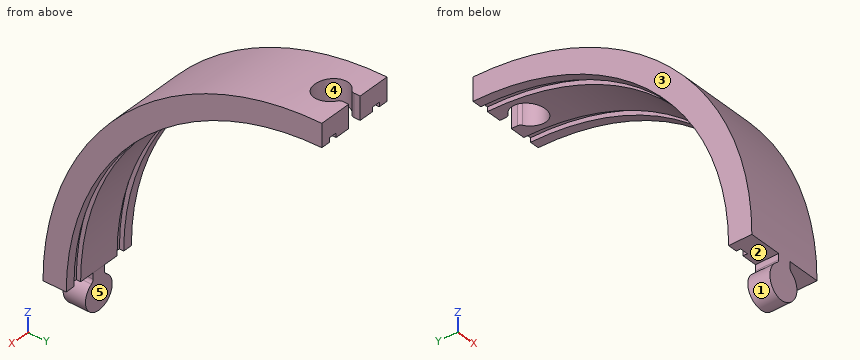
Autodesk Inventor part; units mm, degrees
ref_plane "YZ Plane" through (0, 0, 0) normal (1, 0, 0) x (0, 1, 0)
ref_plane "XZ Plane" through (0, 0, 0) normal (0, 1, 0) x (-1, 0, 0)
ref_plane "XY Plane" through (0, 0, 0) normal (0, 0, 1) x (1, 0, 0)
sketch "Track sketch" plane through (0, 0, 0) normal (0, 0, 1) x (1, 0, 0)
  line L0 (0, 0) -> (86.36, 0)
  line L1 (86.36, 0) -> (86.36, 25.4)
  line L2 (0, 25.4) -> (0, 0)
  line L3 (19.05, 25.4) -> (19.05, 20.6375)
  line L4 (19.05, 20.6375) -> (10.16, 20.6375)
  line L5 (10.16, 20.6375) -> (10.16, 25.4)
  line L6 (43.18, 25.4) -> (43.18, 0) construction
  line L7 (67.31, 25.4) -> (67.31, 20.6375)
  line L8 (67.31, 20.6375) -> (76.2, 20.6375)
  line L9 (76.2, 20.6375) -> (76.2, 25.4)
  line L10 (10.16, 25.4) -> (0, 25.4)
  line L11 (86.36, 25.4) -> (76.2, 25.4)
  line L12 (67.31, 25.4) -> (19.05, 25.4)
  line L13 (0, 0) -> (0, 304.8) construction
  line L14 (0, 304.8) -> (86.36, 304.8) construction
  line L15 (0, 0) -> (0, -25.4)
  line L16 (0, -25.4) -> (86.36, -25.4)
  line L17 (86.36, -25.4) -> (86.36, 0)
  dimension "d0" = 86.36
  dimension "d1" = 25.4
  dimension "d2" = 19.05
  dimension "d3" = 10.16
  dimension "d6" = 4.7625
  dimension "d23" = 304.8
  dimension "d47" = 25.4
revolve "Revolution1" add sketch "Track sketch" angle 90 about axis through (0, 304.8, 0) along (-1, 0, 0) contours L2 L10 L5 L4 L3 L12 L7 L8 L9 L11 L1 L0
sketch "Sketch3" plane through (0, 0, 0) normal (0, 1, 0) x (-1, 0, 0)
  line L0 (-19.50225, 0) -> (-66.85775, 0)
  line L1 (-43.18, 304.8) -> (-43.18, 0) construction
  line L2 (-43.18, 0) -> (-43.18, -37.562444) construction
  arc A0 (-52.968989, -10.557355) -> (-33.391011, -10.557355) centre (-43.18, -25.4) ccw
  line L3 (-50.8, 0) -> (-35.56, 0)
  line L4 (-35.56, 0) -> (-35.56, -6.528638)
  line L5 (-35.56, -9.335629) -> (-50.8, -9.335629) construction
  line L6 (-50.8, -6.528638) -> (-50.8, 0)
  arc A1 (-52.968989, -10.557355) -> (-50.8, -6.528638) centre (-55.626, -6.528638) ccw
  arc A2 (-35.56, -6.528638) -> (-33.391011, -10.557355) centre (-30.734, -6.528638) ccw
  line L7 (0, 0) -> (-86.36, 0)
  line L8 (-86.36, 0) -> (-86.36, 304.8)
  line L9 (0, 304.8) -> (-86.36, 304.8)
  line L10 (0, 0) -> (0, 304.8)
  line L11 (0, 0) -> (-86.36, 0)
  line L12 (0, 304.8) -> (-86.36, 304.8) construction
  line L13 (-43.18, 304.8) -> (-43.18, 65.498651) construction
  point P0 (-43.18, 279.4)
  dimension "d25" = 279.4
  dimension "d26" = 35.56
  dimension "d27" = 25.4
  dimension "d28" = 15.24
  dimension "d29" = 4.826
  dimension "d32" = 86.36
  dimension "d33" = 43.18
  dimension "d34" = 43.18
  dimension "d35" = 25.4
extrude "Extrusion4" add sketch "Sketch3" along normal blind 25.4 contours L4 A2 A0 A1 L6 L0
ref_plane "Work Plane1" through (0, 304.8, 304.8) normal (0, 0, 1) x (1, 0, 0)
sketch "Sketch4" plane through (0, 304.8, 304.8) normal (0, 0, 1) x (1, 0, 0)
  line L0 (0, -304.8) -> (35.56, -304.8)
  line L1 (35.56, -304.8) -> (50.8, -304.8)
  line L2 (50.8, -304.8) -> (86.36, -304.8)
  line L3 (86.36, -304.8) -> (86.36, 0)
  line L4 (0, 0) -> (86.36, 0)
  line L5 (0, -304.8) -> (0, 0)
  line L6 (67.31, 0) -> (19.05, 0)
  line L7 (43.18, 304.8) -> (43.18, 0) construction
  line L8 (43.18, 0) -> (43.18, -37.562444) construction
  arc A0 (33.391011, -10.557355) -> (52.968989, -10.557355) centre (43.18, -25.4) ccw
  line L9 (35.56, 0) -> (50.8, 0)
  line L10 (50.8, 0) -> (50.8, -6.528638)
  line L11 (50.8, -9.335629) -> (35.56, -9.335629) construction
  line L12 (35.56, -6.528638) -> (35.56, 0)
  arc A1 (33.391011, -10.557355) -> (35.56, -6.528638) centre (30.734, -6.528638) ccw
  arc A2 (50.8, -6.528638) -> (52.968989, -10.557355) centre (55.626, -6.528638) ccw
  point P0 (43.18, 279.4)
  dimension "d38" = 279.4
  dimension "d39" = 35.56
  dimension "d40" = 25.4
  dimension "d41" = 15.24
  dimension "d42" = 4.826
  dimension "d43" = 43.18
  dimension "d44" = 25.4
extrude "Extrusion5" cut sketch "Sketch4" against normal blind 50.8 contours L4 L10 A2 A0 A1 L12
sketch "Track sketch outline for Revolution2" plane through (0, 0, 0) normal (0, 0, 1) x (1, 0, 0)
  line L0 (86.36, 0) -> (0, 0)
  line L1 (86.36, -25.4) -> (86.36, 0)
  line L2 (0, -25.4) -> (86.36, -25.4)
  line L3 (0, 0) -> (0, -25.4)
revolve "Revolution2" cut sketch "Track sketch outline for Revolution2" angle 360 about axis through (0, 304.8, 0) along (1, 0, 0)
properties part number "Caufield_Straight_Track"
Part model, mm, in its own coordinate system. Face numbers are marked on the shaded views. A direction names the side the tool comes from. Coordinates: 2 decimals unless noted, no trailing zeros. Loops run counter-clockwise (first coordinate to the right, second up) from the corner with the lowest first, then second, coordinate; pieces in that order, holes last. Notation, with made-up numbers: (-5, 28.5) - (29, 28.5) arc R11 ccw to (29, 48.5) - close; hole circle Ø11 at (33, 15.25). An arc over 180 degrees is marked (long way). Write each question's results on one line, items separated by ' | '. Start each with the question number.
Q1. Drop flat-ended pins along their axis: pin 1 Ø4 at (x, y) = (52, 33) entering from +Z; pin 2 Ø1 at (x, y) = (18.5, 163) entering from -Z; pin 3 Ø3.5 at (y, z) = (12.5, -4) entering from -X. Give the stop position or say it passes through.
Q2. Two-plate mould, pull along X, no slides. Class the marked faces 3, 4 and 5: +X half, -X half, draft (parallel to the pull), parting line (faces both ways), or undercut.
Q3. Slice it at D-D on x = 43.18. Give the cut face in (y, z), and give its area (3 significant figures).
Q4. Slice it at B-B on z = 152. Give the cut face in (x, y), and give its area (3 significant figures).
Q5. Probe line 1 along X through (y, z) = (279.4, 291); line 2 along Y through (x, z) = (28.5, 26.5); line 3 along Z through (x, y) = (69, 274). List the from-to ranges inside material, lowest first.
Q6. Which spindle directions (+Z, -Z, +X, -X, +Y, -Y) get a long thin tool onto all of the face, cutting with end or side? Do the marked faces 1 and 2. Say none if no direction does.
Q7. Slice it at C-C on y = 178. Give the cut face in (x, z), and give its area (3 significant figures).
Q8. Slice it at A-A on y = 265.5. Give the cut face in (x, z).
Answer:
1) pin 1: stops at z = 141.81 | pin 2: stops at z = 245.97 | pin 3: stops at x = 35.56
2) face 3: -X half | face 4: undercut | face 5: draft
3) outline: (3.07, -43.18) - (25.4, -43.18) - (25.4, 0) arc R279.4 cw to (261.62, 276.04) - (261.62, 301.73) arc R304.8 ccw to start | area: 11,600 mm2
4) outline: (0, 40.6) - (86.36, 40.6) - (86.36, 70.36) - (76.2, 70.36) - (76.2, 64.71) - (67.31, 64.71) - (67.31, 70.36) - (19.05, 70.36) - (19.05, 64.71) - (10.16, 64.71) - (10.16, 70.36) - (0, 70.36) - close | area: 2,470 mm2
5) line 1: x = 0 to 25.4, 60.96 to 86.36 | line 2: y = 1.15 to 26.66 | line 3: z = 282.49 to 303.24
6) face 1: +Y, -Y | face 2: -X, +Y, -Y
7) outline: (0, 248.97) - (10.16, 248.97) - (10.16, 254.3) - (19.05, 254.3) - (19.05, 248.97) - (67.31, 248.97) - (67.31, 254.3) - (76.2, 254.3) - (76.2, 248.97) - (86.36, 248.97) - (86.36, 277.17) - (0, 277.17) - close | area: 2,340 mm2
8) outline: (0, 276.62) - (10.16, 276.62) - (10.16, 281.43) - (19.05, 281.43) - (19.05, 276.62) - (32.09, 276.62) - (32.09, 302.26) - (0, 302.26) - close; (54.27, 276.62) - (67.31, 276.62) - (67.31, 281.43) - (76.2, 281.43) - (76.2, 276.62) - (86.36, 276.62) - (86.36, 302.26) - (54.27, 302.26) - close
